Check sheet for the modelled part. Datum: model origin and axes. Units: mm. A direction names the side the tool comes from. Give positions to 0.01 mm unless a question says otherwise; leave off trailing zeros. Write each loop counter-clockwise with the first axis right and the second up, starting at its lowest first coordinate (ties: lowest second). Pieces come first, ordered by that corner, then holes. Notation, with made-up numbers: (-11, 39) -> (20, 39) arc R25 cw to (20, 51) -> close; hole circle Ø3 at (39.25, -29). An arc over 180 degrees is marked (long way). Use a Markdown table: item, result. Add a question column.
1. Cross-section at C-C (y = 132). Enter the section's corners in (x, z), then the cut area to 3 significant figures.
2. Set-up check for faces 5 (the flat face through (-228.275, 438.385, 1.479)), 6 (the flat face through (-2, 846, 0)): record each of +Z, -Z, +X, -X, +Y, -Y from which the full face is reachable in a straight line by a thin tool's end or side.
3. Cross-section at A-A (z = 1.25). Enter the section's corners in (x, y) (3 decimals).
4. Cross-section at B-B (x = 225). Enter the section's corners in (y, z), then the cut area to 3 significant figures.
5. Release check for a two-part mould opening along Y. For faces 1 (the flat face through (-2, 846, 3)), 2 (the flat face through (234.61, 449.36, 1.48)), 3 (the cylindrical face through (524.595, 880.852, 1.479)), 4 (the flat face through (-278.245, 424.935, 1.479)) record: released by +Y, released by -Y, zero draft, split by the parting line, or undercut.
6. Scan lines: probe 1 along Y at (x, z) = (92, 1.8); probe 2 along X at (y, z) = (723, 0.2); probe 3 along X at (y, z) = (761, 2.1). Record each from-to range of solid material in increasing order. Write a range as [from, to].
Autodesk Inventor part; units mm, degrees
ref_plane "YZ Plane" through (0, 0, 0) normal (1, 0, 0) x (0, 1, 0)
ref_plane "XZ Plane" through (0, 0, 0) normal (0, 1, 0) x (-1, 0, 0)
ref_plane "XY Plane" through (0, 0, 0) normal (0, 0, 1) x (1, 0, 0)
sketch "Sketch1" plane through (0, 0, 0) normal (0, 0, 1) x (1, 0, 0)
  circle A0 centre (0, 0) radius 8.5
  line L0 (-524.8067, 851.9919) -> (-24.6817, -14.25)
  arc A1 (-24.6817, -14.25) -> (24.6817, -14.25) centre (0, 0) ccw
  line L1 (24.6817, -14.25) -> (524.8067, 851.9919)
  arc A2 (524.8067, 851.9919) -> (500.125, 894.7419) centre (500.125, 866.2419) ccw
  line L2 (500.125, 894.7419) -> (-500.125, 894.7419)
  arc A3 (-500.125, 894.7419) -> (-524.8067, 851.9919) centre (-500.125, 866.2419) ccw
  line L3 (0, 0) -> (0, 894.7419) construction
  line L4 (-462.8859, 844.7419) -> (462.8859, 844.7419)
  line L5 (462.8859, 844.7419) -> (0, 43)
  line L6 (0, 43) -> (-462.8859, 844.7419)
  circle A4 centre (-500.125, 866.2419) radius 8.5
  circle A5 centre (500.125, 866.2419) radius 8.5
  dimension "d34" = 17
  dimension "d35" = 20
  dimension "d36" = 1000.25
  dimension "d37" = 1000.25
  dimension "d38" = 50
  dimension "d39" = 17
  dimension "d40" = 17
extrude "Plate1" add sketch "Sketch1" along normal blind 3
fillet "Corner Round3" radius 6 3 edges at (-462.8859, 844.7419, 1.5) (0, 43, 1.5) (462.8859, 844.7419, 1.5)
equation "\"d37\" = d36"
equation "\"d2\" = Thickness"
equation "\"BendReliefWidth\" = Thickness"
equation "\"BendReliefDepth\" = 0.5 * Thickness"
equation "\"CornerReliefSize\" = 4 * Thickness"
equation "\"MinimumRemnant\" = 2 * Thickness"
equation "\"TransitionRadius\" = BendRadius"
equation "\"JacobiRadiusSize\" = BendRadius"
equation "\"GapSize\" = Thickness"
properties part number "TZS 1289 leg pattern" material "Stainless Steel"
Worked answers:
| question | item | result |
|---|---|---|
| 1 | outline | (-109.12, 0) -> (-51.38, 0) -> (-51.38, 3) -> (-109.12, 3) -> close; (51.38, 0) -> (109.12, 0) -> (109.12, 3) -> (51.38, 3) -> close |
| 1 | area | 346 mm² |
| 2 | face 5 | +Z, -Z |
| 2 | face 6 | -Z, +X, -X, +Y, -Y |
| 3 | outline | (-524.807, 851.992) -> (-24.682, -14.25) arc R28.5 ccw to (24.682, -14.25) -> (524.807, 851.992) arc R28.5 ccw to (500.125, 894.742) -> (-500.125, 894.742) arc R28.5 ccw to start; hole circle Ø17 at (-500.125, 866.242); hole (-457.69, 835.742) -> (-5.196, 52) arc R6 ccw to (5.196, 52) -> (457.69, 835.742) arc R6 ccw to (452.494, 844.742) -> (-452.494, 844.742) arc R6 ccw to start; hole circle Ø17 at (0, 0); hole circle Ø17 at (500.125, 866.242) |
| 4 | outline | (332.71, 0) -> (432.71, 0) -> (432.71, 3) -> (332.71, 3) -> close; (844.74, 0) -> (894.74, 0) -> (894.74, 3) -> (844.74, 3) -> close |
| 4 | area | 450 mm² |
| 5 | face 1 | zero draft |
| 5 | face 2 | undercut |
| 5 | face 3 | split by the parting line |
| 5 | face 4 | released by -Y |
| 6 | probe 1 | y = [102.35, 202.35], [844.74, 894.74] |
| 6 | probe 2 | x = [-450.33, -392.6], [392.6, 450.33] |
| 6 | probe 3 | x = [-472.27, -414.54], [414.54, 472.27] |
